Geometry check sheet. Reference: the model listing, model coordinates, mm. A direction names the side the tool comes from. Coordinates: 2 decimals unless noted, no trailing zeros. Order: outer loops, then holes, each group sorted by start corner. A loop starts at its lowest first (then second) coordinate and runs counter-clockwise, first axis right, second up. Notation, with made-up numbers: (84.25, 38) - (97.25, 38) arc R20 cw to (97.25, 54) - close; hole circle Ø11 at (32, -31.75). An arc over 180 degrees is marked (long way). Return JSON: item names as keys, results as strings. Group by question number.
Item 1: Section check D-D on x = 2.25. Enter the section's corners in (y, z).
Item 2: Section check C-C on y = -1.5. Enter the section's corners in (x, z).
Item 3: Tool access check on faces 1 (the flat face through (-5, 5, 100)), 2 (the flat face through (-0.14, 0.19, 44.37)), 3 (the flat face through (-4.077, -1.995, 44.37)). Record the directions out of +Z, -Z, +X, -X, +Y, -Y that give a thin tool (end or side, any length) a straight path to the whole face; none if there is none.
Item 4: Section check A-A on z = 71. Enter the section's corners in (x, y).
Item 5: Scan lines: probe 1 along Z at (x, y) = (-1.25, 0); probe 2 along X at (y, z) = (0.5, 76); probe 3 along X at (y, z) = (10.25, 89.5). Record each from-to range of solid material in increasing order.
Item 6: Gauge pin test, flat ends, axial feed: pin 1 (8 mm diameter, centred on x = -10, z = 79, fed in from -Y); pin 2 (3 mm diameter, centred on x = 1, z = 55.5, fed in from +Y); pin 3 (4 mm diameter, centred on x = -0.5, z = 44, fed in from -Y). Record the tip position at first contact, or that the pin passes through.
Item 7: Draft check along X on faces 4 (the flat face through (0.224, 9.861, 44.37)), 5 (the cylindrical face through (-7.517, -4.588, 49.3)), 6 (the flat face through (-5, 3, 0)). Enter one of: pulls with the +X half, pulls with the -X half, needs draft (parallel to the pull), parting line crosses it, or undercut.
Item 8: Section check B-B on x = -11.5. Enter the section's corners in (y, z).
from build123d import *

# Parameters (mm, degrees)
SKETCH_1_R          = 10
EXTRUDE_1_DEPTH     = 100
SKETCH_5_R          = 1.1
CUT_EXTRUDE_3_DEPTH = 4
CUT_EXTRUDE_2_DEPTH = 90


with BuildPart() as part:
    # ｽｹｯﾁ1 → ﾎﾞｽ - 押し出し1 (new body)
    with BuildSketch(Plane.XY):
        with Locations((-5.348947677, 5.174385531)):
            Circle(SKETCH_1_R)
    extrude(amount=EXTRUDE_1_DEPTH)

    # ｽｹｯﾁ5 → ｶｯﾄ - 押し出し3 (cut)
    with BuildSketch(Plane(origin=(0, 0, 0), x_dir=(-1, 0, 0), z_dir=(0, 0, -1))):
        with Locations((5.348947677, 5.174385531)):
            Circle(SKETCH_5_R)
    extrude(amount=-CUT_EXTRUDE_3_DEPTH, mode=Mode.SUBTRACT)

    # ｽｹｯﾁ3 → ｶｯﾄ - 押し出し2 (cut)
    with BuildSketch(Plane(origin=(0, 0, 0), x_dir=(-1, 0, 0), z_dir=(0, 0, -1))):
        Polygon((9.180368817, 6.810812261), (9.286390444, 3.812686278), (9.339401258, 2.313623286), (15.282642412, 4.024729531), (17.281393068, 4.095410616), (17.175371441, 7.093536599), (15.176620785, 7.022855515), (9.127358004, 8.309875253), align=None)
        Polygon((2.016049987, 7.674280205), (4.559492439, 9.265160619), (5.831213665, 10.060600826), (1.377731611, 14.352045524), (0.317144668, 16.047673826), (-2.226297784, 14.456793412), (-1.165710841, 12.76116511), (0.74432876, 6.878839998), align=None)
        Polygon((4.850424227, 1.038064125), (2.200960148, 2.445309695), (0.876228108, 3.14893248), (-0.613530992, -2.853618463), (-1.551694705, -4.619927849), (1.097769374, -6.027173419), (2.035933088, -4.260864033), (6.175156267, 0.33444134), align=None)
    extrude(amount=-CUT_EXTRUDE_2_DEPTH, mode=Mode.SUBTRACT)


solid = part.part
Computed:
{
 "1": {"outline": "(-1.33, 0) - (11.67, 0) - (11.67, 100) - (-1.33, 100) - close"},
 "2": {"outline": "(-12.8, 0) - (-4.52, 0) - (-4.52, 90) - (0.28, 90) - (0.28, 0) - (2.1, 0) - (2.1, 100) - (-12.8, 100) - close"},
 "3": {"face 1": "+Z, +X, -X, +Y, -Y", "face 2": "-Z, -Y", "face 3": "-Z"},
 "4": {"outline": "(-15.28, 4.02) arc R10 ccw to (-2.04, -4.26) - (-6.18, 0.33) - (-0.88, 3.15) - (0.61, -2.85) arc R10 ccw to (1.17, 12.76) - (-0.74, 6.88) - (-5.83, 10.06) - (-1.38, 14.35) arc R10 ccw to (-15.18, 7.02) - (-9.13, 8.31) - (-9.34, 2.31) - close"},
 "5": {"probe 1": "z = 90 to 100", "probe 2": "x = -14.19 to -5.86, -0.22 to 3.49", "probe 3": "x = -13.97 to -5.63, 0.35 to 3.27"},
 "6": {"pin 1": "stops at y = -4.8", "pin 2": "stops at y = 12.76", "pin 3": "stops at y = -4.41"},
 "7": {"face 4": "undercut", "face 5": "parting line crosses it", "face 6": "needs draft"},
 "8": {"outline": "(-2.71, 0) - (2.94, 0) - (2.94, 90) - (7.81, 90) - (7.81, 0) - (13.06, 0) - (13.06, 100) - (-2.71, 100) - close"}
}
